Input: part model. Units: mm. Frame: model coordinates. A direction names the side the tool comes from. Give positions to 0.01 mm unless a question says otherwise; leave off trailing zeros. Loops run counter-clockwise (first coordinate to the right, second up) from the corner with the lowest first, then second, coordinate; pieces in that order, holes last. Notation, with made-up numbers: (14.25, 65.5) -> (47.25, 65.5) arc R17 ccw to (47.25, 71.5) -> close; hole circle Ø1 at (49.25, 38.5). An arc over 180 degrees is marked (long way). Answer as a JSON object with one key per item and string values.
```python
from build123d import *

# Parameters (mm, degrees)
EXTRUDE_THIN1_DEPTH = 19
CUT_EXTRUDE1_DEPTH  = 4
CUT_EXTRUDE2_DEPTH  = 10


with BuildPart() as part:
    # Sketch2 → Extrude-Thin1 (new body, symmetric)
    with BuildSketch(Plane.XY):
        Polygon((-1.5, 32), (-1.5, -1.5), (63, -1.5), (63, 1.5), (1.5, 1.5), (1.5, 32), align=None)
    extrude(amount=EXTRUDE_THIN1_DEPTH, both=True)

    # Sketch3 → Cut-Extrude1 (cut, through all)
    with BuildSketch(Plane(origin=(1.5, 0, 0), x_dir=(0, 0, -1), z_dir=(1, 0, 0))):
        with BuildLine():
            Line((5, 23.298608028), (12, 23.298608028))
            ThreePointArc((12, 23.298608028), (15, 20.298608028), (12, 17.298608028))
            Line((12, 17.298608028), (5, 17.298608028))
            ThreePointArc((5, 17.298608028), (2, 20.298608028), (5, 23.298608028))
        make_face()
        with BuildLine():
            Line((-12, 13.03992903), (-5, 13.03992903))
            ThreePointArc((-5, 13.03992903), (-2, 10.03992903), (-5, 7.03992903))
            Line((-5, 7.03992903), (-12, 7.03992903))
            ThreePointArc((-12, 7.03992903), (-15, 10.03992903), (-12, 13.03992903))
        make_face()
        with BuildLine():
            Line((-15.496537692, 27.749610789), (15.496537692, 27.749610789))
            ThreePointArc((15.496537692, 27.749610789), (17.973859648, 26.723470437), (19, 24.246148481))
            Line((19, 24.246148481), (19, 32))
            Line((19, 32), (-19, 32))
            Line((-19, 32), (-19, 24.246148481))
            ThreePointArc((-19, 24.246148481), (-17.973859648, 26.723470437), (-15.496537692, 27.749610789))
        make_face()
    extrude(amount=-CUT_EXTRUDE1_DEPTH, mode=Mode.SUBTRACT)

    # Sketch4 → Cut-Extrude2 (cut)
    with BuildSketch(Plane(origin=(0, 1.5, 0), x_dir=(1, 0, 0), z_dir=(0, 1, 0))):
        with BuildLine():
            Line((42.625671961, -14.5), (23.625671961, -14.5))
            ThreePointArc((23.625671961, -14.5), (9.125671961, 0), (23.625671961, 14.5))
            Line((23.625671961, 14.5), (42.625671961, 14.5))
            ThreePointArc((42.625671961, 14.5), (57.125671961, 0), (42.625671961, -14.5))
        make_face()
        with BuildLine():
            Line((42.625671961, 19), (63, 19))
            Line((63, 19), (63, -19))
            Line((63, -19), (42.625671961, -19))
            ThreePointArc((42.625671961, -19), (61.625671961, 0), (42.625671961, 19))
        make_face()
    extrude(amount=-CUT_EXTRUDE2_DEPTH, mode=Mode.SUBTRACT)


solid = part.part
```
Q1. Ray query, line 1 along X through (y, z) = (26.5, 3). Return the intervals inside material, ascending.
Evaluation:
{"line 1": "x = -1.5 to 1.5"}
Q2. Section D-D, the plane y = 9. Return the cut outline in (x, z).
Evaluation:
{"outline": "(-1.5, -19) -> (1.5, -19) -> (1.5, 2.19) -> (-1.5, 2.19) -> close; (-1.5, 14.81) -> (1.5, 14.81) -> (1.5, 19) -> (-1.5, 19) -> close"}
Q3. Draft query along Y for faces 4 (the flat face through (8.6, -1.5, 0.3)), 5 (the flat face through (0, 17.299, -9)), 6 (the flat face through (-1.5, 13, 0)). Return one class per face: +Y half, -Y half, draft (parallel to the pull), parting line (faces both ways), or undercut.
Evaluation:
{"face 4": "-Y half", "face 5": "undercut", "face 6": "draft"}
Q4. Pin query (flat end, axial travel): pin 1 (19 mm diameter, centred on x = 27, z = -5.5, fed in from +Y); pin 2 (4 mm diameter, centred on y = 2, z = 3.5, fed in from +X); pin 3 (13 mm diameter, centred on y = 17, z = 4, fed in from +X). Return the tip coordinate at first contact, or that it passes through.
Evaluation:
{"pin 1": "stops at y = 1.5", "pin 2": "stops at x = 61.56", "pin 3": "stops at x = 1.5"}
Q5. Access query for faces 1 (the flat face through (1.5, 14, 0)), 2 (the flat face through (33, 0, -14.5)), 3 (the cylindrical face through (0, 20.2, -2)). Directions: +Z, -Z, +X, -X, +Y, -Y. A direction counts if a zero-diameter tool reaches every point of the face in a straight line with its end or side. Return the directions, or none.
Evaluation:
{"face 1": "+Z, -Z, +X, +Y", "face 2": "+Y, -Y", "face 3": "+X, -X"}
Q6. Section C-C, the plane z = -4. Return the cut outline in (x, y), then the cut area to 3 significant figures.
Evaluation:
{"outline": "(-1.5, -1.5) -> (9.69, -1.5) -> (9.69, 1.5) -> (1.5, 1.5) -> (1.5, 17.47) -> (-1.5, 17.47) -> close; (-1.5, 23.13) -> (1.5, 23.13) -> (1.5, 27.75) -> (-1.5, 27.75) -> close; (56.56, -1.5) -> (61.2, -1.5) -> (61.2, 1.5) -> (56.56, 1.5) -> close", "area": "109 mm2"}
Q7. Section A-A, the plane z = 0. Return the cut outline in (x, y).
Evaluation:
{"outline": "(-1.5, -1.5) -> (9.13, -1.5) -> (9.13, 1.5) -> (1.5, 1.5) -> (1.5, 27.75) -> (-1.5, 27.75) -> close; (57.13, -1.5) -> (61.63, -1.5) -> (61.63, 1.5) -> (57.13, 1.5) -> close"}
Q8. Section B-B, the plane x = 37. Return the cut outline in (y, z).
Evaluation:
{"outline": "(-1.5, -19) -> (1.5, -19) -> (1.5, -14.5) -> (-1.5, -14.5) -> close; (-1.5, 14.5) -> (1.5, 14.5) -> (1.5, 19) -> (-1.5, 19) -> close"}
